from build123d import *

# Parameters (mm, degrees)
F0_W      = 420
F0_H      = 420
F1_DEPTH  = 105
F2_T      = -6
F3_W      = 6
F3_H      = 408
F4_DEPTH  = 18
F5_W      = 6
F5_H      = 408
F6_DEPTH  = 18
F7_W      = 6
F7_H      = 18
F8_DEPTH  = 372
F9_W      = 6
F9_H      = 18
F10_DEPTH = 372
F11_W     = 408
F11_H     = 408
F11_W_2   = 400
F11_H_2   = 400
F12_DEPTH = 10
F14_W     = 400
F14_H     = 400
F15_DEPTH = 10
F16_DEPTH = 25.4
F18_DEPTH = 25.4


with BuildPart() as f1:
    # F0 (on Front) → F1 (new body, symmetric)
    with BuildSketch(Plane.XZ):
        Rectangle(F0_W, F0_H)
    extrude(amount=F1_DEPTH, both=True)

    # F2
    f2_openings = [f1.faces().sort_by_distance(p)[0] for p in [
        (0, -105, 0),
    ]]
    offset(amount=F2_T, openings=f2_openings)

    # F3 (on face) → F4 (join)
    with BuildSketch(Plane.YZ.offset(-204)):
        with Locations((-92, 0)):
            Rectangle(F3_W, F3_H)
    extrude(amount=F4_DEPTH)

    # F5 (on face) → F6 (join)
    with BuildSketch(Plane(origin=(204, 0, 0), x_dir=(0, -1, 0), z_dir=(-1, 0, 0))):
        with Locations((92, 0)):
            Rectangle(F5_W, F5_H)
    extrude(amount=F6_DEPTH)

    # F7 (on face) → F8 (join, through all)
    with BuildSketch(Plane.YZ.offset(-186)):
        with Locations((-92, 195)):
            Rectangle(F7_W, F7_H)
    extrude(amount=F8_DEPTH)

    # F9 (on face) → F10 (join, through all)
    with BuildSketch(Plane.YZ.offset(-186)):
        with Locations((-92, -195)):
            Rectangle(F9_W, F9_H)
    extrude(amount=F10_DEPTH)

    # F11 (on face) → F12 (join)
    with BuildSketch(Plane.XZ.offset(95)):
        Rectangle(F11_W, F11_H)
        Rectangle(F11_W_2, F11_H_2, mode=Mode.SUBTRACT)
    extrude(amount=F12_DEPTH)

    # F13: F1 across face


with BuildPart() as f1_1:
    add(f1.part)
    add(f1.part.mirror(Plane(origin=(0, 0, -210), x_dir=(1, 0, 0), z_dir=(0, 0, -1))))

    # F14 (on face) → F15 (join)
    with BuildSketch(Plane.XZ.offset(95)):
        with Locations((0, -420)):
            Rectangle(F14_W, F14_H)
    extrude(amount=F15_DEPTH)

    # F16 (cut): a face of the model
    f16_faces = [f1_1.faces().sort_by_distance(p)[0] for p in [
        (0, 5, -204),
    ]]
    extrude(f16_faces, amount=-F16_DEPTH, mode=Mode.SUBTRACT)

    # F17: F1 across face


with BuildPart() as f1_2:
    add(f1_1.part)
    add(f1_1.part.mirror(Plane(origin=(210, 0, -210), x_dir=(0, 1, 0), z_dir=(1, 0, 0))))

    # F18 (cut): a face of the model
    f18_faces = [f1_2.faces().sort_by_distance(p)[0] for p in [
        (216, 5, -210),
    ]]
    extrude(f18_faces, amount=-F18_DEPTH, mode=Mode.SUBTRACT)


solid = f1_2.part
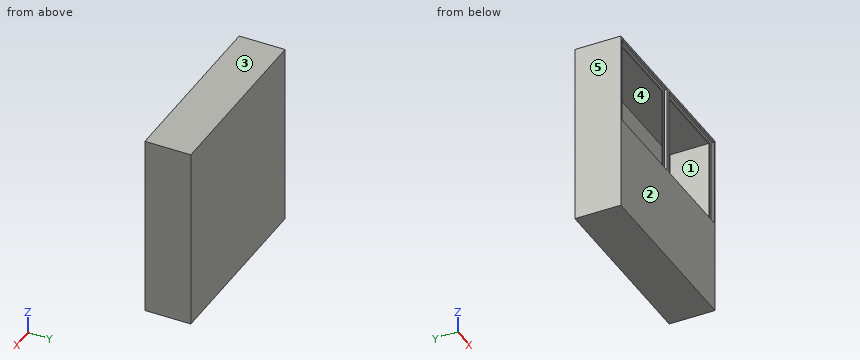
Verification items for the finished model (mm, model axes). Face numbers are marked on the shaded views. A direction names the side the tool comes from. Give positions to 0.01 mm unless a question says otherwise; leave off trailing zeros. Write each loop counter-clockwise with the first axis right and the second up, starting at its lowest first coordinate (ties: lowest second). Pieces come first, ordered by that corner, then holes.
(1) Cross-section at D-D (x = -130.5). Enter the section's corners in (y, z).
(2) Access from +Z, -Z, +X, -X, +Y, -Y to the whole of each face (thin tool, end or side, straight path). Record for the marked faces 4 and 5.
(3) Cross-section at C-C (y = -38). Enter the section's corners in (x, z).
(4) Material ranges on line 1 (X direction, y = -95.5, z = 38); line 2 (X direction, y = -91, z = -401); line 3 (Y direction, x = 191.5, z = -464.5), recorded low to high.
(5) Cross-section at B-B (z = -23.5). Enter the section's corners in (x, y).
(6) Cross-section at A-A (z = -487). Enter the section's corners in (x, y), plus the area to 3 significant figures.
(7) Mould release check, pull along Z, two halves, no side actions. Record for the marked faces 1, 2 and 3: +Z half, -Z half, draft (parallel to the pull), parting line (faces both ways), or undercut.
(8) Gauge pin test, flat end, axial feed: pin 1 (5 mm diameter, centred on x = 113.5, z = -136, fed in from -Y). Record the tip position at first contact, or that the pin passes through.
Worked out:
1. outline: (-105, -630) - (105, -630) - (105, 210) - (-105, 210) - (-105, 200) - (-95, 200) - (-95, 186) - (-89, 186) - (-89, 204) - (99, 204) - (99, -624) - (-89, -624) - (-89, -606) - (-95, -606) - (-95, -234) - (-89, -234) - (-89, -186) - (-95, -186) - (-95, -200) - (-105, -200) - close
2. face 4: none
2. face 5: +Z, -Z, -X, +Y, -Y
3. outline: (-210, -630) - (630, -630) - (630, 210) - (-210, 210) - close; hole (-204, -624) - (624, -624) - (624, 204) - (-204, 204) - close
4. line 1: x = -210 to -200, 200 to 220, 620 to 630
4. line 2: x = -210 to -186, 186 to 234, 606 to 630
4. line 3: y = -105 to -89, 99 to 105
5. outline: (-210, -105) - (-200, -105) - (-200, -95) - (-186, -95) - (-186, -89) - (-204, -89) - (-204, 99) - (624, 99) - (624, -89) - (606, -89) - (606, -95) - (620, -95) - (620, -105) - (630, -105) - (630, 105) - (-210, 105) - close; (186, -95) - (200, -95) - (200, -105) - (220, -105) - (220, -95) - (234, -95) - (234, -89) - (186, -89) - close
6. outline: (-210, -105) - (630, -105) - (630, 105) - (-210, 105) - close; hole (-204, -89) - (-186, -89) - (-186, -95) - (186, -95) - (186, -89) - (234, -89) - (234, -95) - (606, -95) - (606, -89) - (624, -89) - (624, 99) - (-204, 99) - close
6. area: 16,300 mm2
7. face 1: undercut
7. face 2: draft
7. face 3: +Z half
8. pin 1: stops at y = 99
